For this review, take the finished solid that the model builds, in its own axes (mm). A direction names the side the tool comes from. Coordinates: 2 decimals unless noted, no trailing zeros. Order: outer loops, then holes, each group sorted by start corner. A loop starts at its lowest first (then second) coordinate and runs counter-clockwise, first axis right, second up. Notation, with made-up numbers: (59.5, 25) -> (111.5, 25) arc R18 ccw to (111.5, 55) -> close; hole circle Ø7 at (57, -0.75). An arc over 180 degrees is marked (long way). Answer as a JSON object with one key per item and string values. Group by question number.
1) Add section A-A, the plane z = 39. Write out the cut boundary in (x, y), then the cut area to 3 significant figures.
2) Draft analysis for pull direction Y (two halves, no side actions). For faces 1 (the cylindrical face through (-4.51, 2.16, 58.99)), 2 (the flat face through (14, 12, 34.5)), 3 (the cylindrical face through (-13.267, -12.165, 47.428)), state which applies: +Y half, -Y half, draft (parallel to the pull), parting line (faces both ways), or undercut.
3) Wall thickness on L1, parallel to Z at x = -5, y = -16.5; L2, parallel to Y at x = -0.5, z = 41.5; L3, parallel to Z at x = -14, y = -4.5: over which ranges is each line inside the solid? List them lowest first.
4) Machinability: for faces 4 (the cylindrical face through (-10.316, 7.91, 0.986)), 5 (the flat face through (-4, 4, 58)), 6 (the cylindrical face through (0, -5, 59)), which of the approach directions +Z, -Z, +X, -X, +Y, -Y give a long, thin tool a straight path to every point of the face, cutting with its end or side? Answer none if there is none.
5) For pin 1 (13 mm diameter, centred on x = 4.5, y = 3.5, fed in from -Z); pin 2 (5 mm diameter, centred on x = 8.5, z = 28.5, fed in from +Y); pin 3 (0.8 mm diameter, centred on x = 0, z = 32.5, fed in from +Y), all flat-tipped, find the tip position at first contact; note any pin that passes through.
from build123d import *

# Parameters (mm, degrees)
SKETCH1_W          = 3.5
SKETCH1_H          = 5
CUT_EXTRUDE1_DEPTH = 2
SKETCH3_5_R        = 17
CUT_EXTRUDE2_DEPTH = 1
CUT_EXTRUDE3_START = -2
SKETCH5_R          = 5
SKETCH5_R_2        = 2
CUT_EXTRUDE3_DEPTH = 2


with BuildPart() as part:
    # Sketch1 → Revolve1 (revolve)
    with BuildSketch(Plane(origin=(0, 0, 0), x_dir=(0, 0, -1), z_dir=(1, 0, 0)), mode=Mode.PRIVATE) as revolve1_sk:
        Polygon((-60, 18), (-60, 5), (-58, 5), (-58, 17), (-31, 17), (-31, 18), (-34.5, 18), align=None)
        with Locations((-32.75, 20.5)):
            Rectangle(SKETCH1_W, SKETCH1_H)
        with Locations((-29.25, 20.5)):
            Rectangle(SKETCH1_W, SKETCH1_H)
        Polygon((-31, 18), (-31, 17), (-2, 17), (-2, 13), (0, 13), (0, 18), (-27.5, 18), align=None)
    revolve(revolve1_sk.sketch.rotate(Axis((0, 0, 1072.381477522), (0, 0, -1)), 90), axis=Axis((0, 0, 1072.381477522), (0, 0, -1)))

    # Sketch3 → Cut-Extrude1 (cut, symmetric)
    with BuildSketch(Plane.XY.offset(31)):
        with BuildLine():
            ThreePointArc((-6.498382723, 17.854159795), (0, -19), (6.498382723, 17.854159795))
            Line((6.498382723, 17.854159795), (7.524443153, 20.673237657))
            ThreePointArc((7.524443153, 20.673237657), (0, 22), (-7.524443153, 20.673237657))
            Line((-7.524443153, 20.673237657), (-6.498382723, 17.854159795))
        make_face()
        with BuildLine():
            add(Edge.make_bspline(
                [(-1, 19.972475891), (-1.837517439, 19.972475891), (-3.400702548, 17.606617047), (-4.505243001, 16.51810785)],
                knots=[0, 0, 0, 0, 1, 1, 1, 1], degree=3))
            Line((-1, 19.972475891), (1, 19.972475891))
            add(Edge.make_bspline(
                [(1, 19.972475891), (1.837517439, 19.972475891), (3.400702548, 17.606617047), (4.505243001, 16.51810785)],
                knots=[0, 0, 0, 0, 1, 1, 1, 1], degree=3))
            Line((4.505243001, 16.51810785), (4.683957663, 16.341987046))
            ThreePointArc((4.683957663, 16.341987046), (13.576215973, 10.231635249), (17, 0))
            ThreePointArc((17, 0), (-10.231635249, -13.576215973), (-4.683957663, 16.341987046))
            Line((-4.683957663, 16.341987046), (-4.505243001, 16.51810785))
        make_face(mode=Mode.SUBTRACT)
    extrude(amount=CUT_EXTRUDE1_DEPTH, both=True, mode=Mode.SUBTRACT)

    # Sketch3<5> → Cut-Extrude2 (cut, symmetric)
    with BuildSketch(Plane.XY.offset(31)):
        Circle(SKETCH3_5_R)
        with BuildLine():
            Line((1, 19.972475891), (-1, 19.972475891))
            add(Edge.make_bspline(
                [(-1, 19.972475891), (-1.837517439, 19.972475891), (-3.400702548, 17.606617047), (-4.505243001, 16.51810785)],
                knots=[0, 0, 0, 0, 1, 1, 1, 1], degree=3))
            Line((-4.505243001, 16.51810785), (-4.683957663, 16.341987046))
            ThreePointArc((-4.683957663, 16.341987046), (0, 17), (4.683957663, 16.341987046))
            Line((4.683957663, 16.341987046), (4.505243001, 16.51810785))
            add(Edge.make_bspline(
                [(1, 19.972475891), (1.837517439, 19.972475891), (3.400702548, 17.606617047), (4.505243001, 16.51810785)],
                knots=[0, 0, 0, 0, 1, 1, 1, 1], degree=3))
        make_face()
        with BuildLine():
            Line((7.524443153, 20.673237657), (6.498382723, 17.854159795))
            ThreePointArc((6.498382723, 17.854159795), (0, -19), (-6.498382723, 17.854159795))
            Line((-6.498382723, 17.854159795), (-7.524443153, 20.673237657))
            ThreePointArc((-7.524443153, 20.673237657), (-12.6186816, -18.021344974), (22, 0))
            ThreePointArc((22, 0), (18.021344974, 12.6186816), (7.524443153, 20.673237657))
        make_face()
    extrude(amount=CUT_EXTRUDE2_DEPTH, both=True, mode=Mode.SUBTRACT)

    # Sketch5 → Cut-Extrude3 (cut)
    with BuildSketch(Plane.XY.offset(60).offset(CUT_EXTRUDE3_START)):
        Circle(SKETCH5_R)
        with Locations((-3.830222216, -3.213938048)):
            Circle(SKETCH5_R_2)
        with Locations((0, 5)):
            Circle(SKETCH5_R_2)
        with Locations((3.830222216, -3.213938048)):
            Circle(SKETCH5_R_2)
    extrude(amount=CUT_EXTRUDE3_DEPTH, mode=Mode.SUBTRACT)


solid = part.part
Output values:
{
 "1": {"outline": "circle Ø36 at (0, 0); hole circle Ø34 at (0, 0)", "area": "110 mm²"},
 "2": {"face 1": "undercut", "face 2": "draft", "face 3": "parting line"},
 "3": {"L1": "z = 0 to 29, 33 to 60", "L2": "y = -17.99 to -16.99, 16.99 to 17.99", "L3": "z = 0 to 2, 58 to 60"},
 "4": {"face 4": "-Z", "face 5": "none", "face 6": "+Z, -Z"},
 "5": {"pin 1": "stops at z = 58", "pin 2": "stops at y = 22.2", "pin 3": "stops at y = 23"}
}
